```python
from build123d import *

# Parameters (mm, degrees)
BOSS_EXTRUDE1_DEPTH = 3.175
FILLET1_R           = 5.08
SKETCH2_R           = 2.413
SKETCH2_W           = 25.4
SKETCH2_H           = 12.7
CUT_EXTRUDE1_DEPTH  = 113.917603541
SKETCH3_W           = 27.94
SKETCH3_H           = 50.8
CUT_EXTRUDE2_DEPTH  = 113.917603541


with BuildPart() as part:
    # Sketch1 → Boss-Extrude1 (new body)
    with BuildSketch(Plane(origin=(0, 0, 0), x_dir=(1, 0, 0), z_dir=(0, 1, 0))):
        Polygon((25.4, 50.8), (49.170566038, 50.8), (49.170566038, 101.6), (-27.029433962, 101.6), (-27.029433962, 50.8), (0, 50.8), (0, 0), (25.4, 0), align=None)
    extrude(amount=BOSS_EXTRUDE1_DEPTH)

    # Fillet1
    fillet1_edges = [part.edges().sort_by_distance(p)[0] for p in [
        (-27.029433962, 1.5875, -50.8),
        (-27.029433962, 1.5875, -101.6),
        (49.170566038, 1.5875, -101.6),
        (49.170566038, 1.5875, -50.8),
        (25.4, 1.5875, 0),
        (0, 1.5875, 0),
    ]]
    fillet(fillet1_edges, radius=FILLET1_R)

    # Sketch2 → Cut-Extrude1 (cut, through all)
    with BuildSketch(Plane(origin=(0, 3.175, 0), x_dir=(1, 0, 0), z_dir=(0, 1, 0))):
        with Locations(Location((12.7, 19.05, 0), (0, 0, 270))):
            Circle(SKETCH2_R)
        with Locations(Location((12.7, 31.75, 0), (0, 0, 270))):
            Circle(SKETCH2_R)
        with Locations(Location((12.7, 44.45, 0), (0, 0, 270))):
            Circle(SKETCH2_R)
        with Locations(Location((-12.698753962, 88.9, 0), (0, 0, 270))):
            Circle(SKETCH2_R)
        with Locations(Location((0.001246038, 88.9, 0), (0, 0, 270))):
            Circle(SKETCH2_R)
        with Locations(Location((12.701246038, 88.9, 0), (0, 0, 270))):
            Circle(SKETCH2_R)
        with Locations(Location((25.401246038, 88.9, 0), (0, 0, 270))):
            Circle(SKETCH2_R)
        with Locations(Location((38.101246038, 88.9, 0), (0, 0, 270))):
            Circle(SKETCH2_R)
        with Locations(Location((12.701246038, 63.5, 0), (0, 0, 270))):
            Circle(SKETCH2_R)
        with Locations(Location((25.401246038, 63.5, 0), (0, 0, 270))):
            Circle(SKETCH2_R)
        with Locations(Location((38.101246038, 63.5, 0), (0, 0, 270))):
            Circle(SKETCH2_R)
        with Locations((12.7, 6.35)):
            Rectangle(SKETCH2_W, SKETCH2_H)
    extrude(amount=-CUT_EXTRUDE1_DEPTH, mode=Mode.SUBTRACT)

    # Sketch3 → Cut-Extrude2 (cut, through all)
    with BuildSketch(Plane(origin=(0, 3.175, 0), x_dir=(1, 0, 0), z_dir=(0, 1, 0))):
        with Locations((-13.97, 76.2)):
            Rectangle(SKETCH3_W, SKETCH3_H)
    extrude(amount=-CUT_EXTRUDE2_DEPTH, mode=Mode.SUBTRACT)


solid = part.part
```
The model under review builds one solid part; all positions refer to its coordinate system, in mm. A direction names the side the tool comes from. Round coordinates to 2 decimals unless told otherwise and drop trailing zeros. Loops run counter-clockwise (first coordinate to the right, second up) from the corner with the lowest first, then second, coordinate; pieces in that order, holes last. Notation, with made-up numbers: (-2.5, 80) - (25.5, 80) arc R18 ccw to (25.5, 94) - close; hole circle Ø4 at (32.25, -34). An arc over 180 degrees is marked (long way). Use a Markdown table: item, result. Add a question column.
Q1. Add section D-D (y = 0.8). State how many separate pieces and enclosed holes the cut face has, plus the area to 3 significant figures.
Q2. Insertion check: pin 1 Ø4 at (x, z) = (25.4, -88.9) entering from -Y; pin 2 Ø1.5 at (x, y) = (31.5, 2.5) entering from +Z; pin 3 Ø6.5 at (x, z) = (38.1, -88.9) entering from -Y. Each pin has a flat end and moves straight along its axis. Give the tip position at first contact, or say it passes through.
Q3. For probe 1 along X at (y, z) = (1.85, -63.5); probe 2 along X at (y, z) = (1, -88.9); probe 3 along Z at (x, y) = (26, 1.35), list the stretches that pass through material, from the lowest coordinate up.
Q4. Add section B-B (z = -44.45). State the section outline as (x, y) points (3 decimals).
Q5. Machinability: for faces 1 (the face through (19, 0, -68)), 2 (the face through (25.4, 2, -31)), which of the approach directions +Z, -Z, +X, -X, +Y, -Y give a long, thin tool a straight path to every point of the face, cutting with its end or side? Answer none if there is none.
Q6. The part is to be moulded in two halves that separate along X. For faces 3 (the face through (24.48, 1.61, -86.67)), 4 (the face through (10.559, 1.61, -30.637)), 5 (the face through (47.643, 1.61, -52.249)), 6 (the face through (22, 2, -101.6)), say which applies: pulls with the +X half, pulls with the -X half, needs draft (parallel to the pull), parting line crosses it, or undercut.
Q7. Add section A-A (z = -63.5). State the section outline as (x, y) points (3 decimals), plus the area to 3 significant figures.
Q8. Add section C-C (z = -88.9). State the section outline as (x, y) points (3 decimals), plus the area to 3 significant figures.
Worked answers:
| question | item | result |
|---|---|---|
| 1 | separate pieces | 1 |
| 1 | enclosed holes | 9 |
| 1 | area | 3,280 mm² |
| 2 | pin 1 | through |
| 2 | pin 2 | z = -50.8 |
| 2 | pin 3 | y = 0 |
| 3 | probe 1 | 0 to 10.29, 15.11 to 22.99, 27.81 to 35.69, 40.51 to 49.17 |
| 3 | probe 2 | 2.41 to 10.29, 15.11 to 22.99, 27.81 to 35.69, 40.51 to 49.17 |
| 3 | probe 3 | -101.6 to -91.24, -86.56 to -65.84, -61.16 to -50.8 |
| 4 | outline | (0, 0) - (10.287, 0) - (10.287, 3.175) - (0, 3.175) - close; (15.113, 0) - (25.4, 0) - (25.4, 3.175) - (15.113, 3.175) - close |
| 5 | face 1 | +Z, -Z, +X, -X, -Y |
| 5 | face 2 | +Z, +X, +Y, -Y |
| 6 | face 3 | undercut |
| 6 | face 4 | undercut |
| 6 | face 5 | pulls with the +X half |
| 6 | face 6 | needs draft |
| 7 | outline | (0, 0) - (10.288, 0) - (10.288, 3.175) - (0, 3.175) - close; (15.114, 0) - (22.988, 0) - (22.988, 3.175) - (15.114, 3.175) - close; (27.814, 0) - (35.688, 0) - (35.688, 3.175) - (27.814, 3.175) - close; (40.514, 0) - (49.171, 0) - (49.171, 3.175) - (40.514, 3.175) - close |
| 7 | area | 110 mm² |
| 8 | outline | (2.414, 0) - (10.288, 0) - (10.288, 3.175) - (2.414, 3.175) - close; (15.114, 0) - (22.988, 0) - (22.988, 3.175) - (15.114, 3.175) - close; (27.814, 0) - (35.688, 0) - (35.688, 3.175) - (27.814, 3.175) - close; (40.514, 0) - (49.171, 0) - (49.171, 3.175) - (40.514, 3.175) - close |
| 8 | area | 102 mm² |
